Geometry: final body of the model. Coordinates: model frame, mm. A direction names the side the tool comes from. Give positions to 0.01 mm unless a question says otherwise; leave off trailing zeros. Write each loop counter-clockwise with the first axis right and the second up, starting at its lowest first coordinate (ties: lowest second). Pieces come first, ordered by that corner, then holes.
from build123d import *

# Parameters (mm, degrees)
BOSS_EXTRU_1_DEPTH      = 5
BOSS_EXTRU_2_DEPTH      = 5
ESQUISSE3_R             = 4
ENL_V_MAT_EXTRU_1_DEPTH = 5


with BuildPart() as part:
    # Esquisse1 → Boss.-Extru.1 (new body)
    with BuildSketch(Plane.XY):
        with BuildLine():
            Line((16.587839799, 53.843180126), (-35.88556985, 8.175453138))
            ThreePointArc((-35.88556985, 8.175453138), (-31.864665417, -54.486574909), (27.523708309, -34.097398918))
            Line((27.523708309, -34.097398918), (49.496452515, 31.904105008))
            ThreePointArc((49.496452515, 31.904105008), (41.417346329, 55.43644284), (16.587839799, 53.843180126))
        make_face()
        with BuildLine():
            Line((23.152792246, 46.299878504), (-29.320617403, 0.632151516))
            ThreePointArc((-29.320617403, 0.632151516), (-26.31766346, -46.166071962), (18.035678944, -30.938712678))
            Line((18.035678944, -30.938712678), (40.008423149, 35.062791248))
            ThreePointArc((40.008423149, 35.062791248), (35.870344371, 47.115939894), (23.152792246, 46.299878504))
        make_face(mode=Mode.SUBTRACT)
    extrude(amount=BOSS_EXTRU_1_DEPTH)

    # Esquisse2 → Boss.-Extru.2 (add)
    with BuildSketch(Plane.XY.offset(5)):
        with BuildLine():
            Line((16.587839799, 53.843180126), (-35.88556985, 8.175453138))
            ThreePointArc((-35.88556985, 8.175453138), (-31.864665417, -54.486574909), (27.523708309, -34.097398918))
            Line((27.523708309, -34.097398918), (49.496452515, 31.904105008))
            ThreePointArc((49.496452515, 31.904105008), (41.417346329, 55.43644284), (16.587839799, 53.843180126))
        make_face()
    extrude(amount=BOSS_EXTRU_2_DEPTH)

    # Esquisse3 → Enlèv. mat.-Extru.1 (cut)
    with BuildSketch(Plane.XY.offset(10)):
        with Locations((-9.954007684, -21.62058827)):
            Circle(ESQUISSE3_R)
    extrude(amount=-ENL_V_MAT_EXTRU_1_DEPTH, mode=Mode.SUBTRACT)


solid = part.part
Q1. Ray query, line 1 along Y through (x, z) = (14, 3); line 2 along Y through (x, z) = (9.5, 3.25); line 3 along X through (y, z) = (19, 3.75). Return the intervals inside material, ascending.
Filled sheet:
line 1: y = -53.03 to -38.84, 38.33 to 51.59
line 2: y = -56 to -43.8, 34.42 to 47.67
line 3: x = -23.45 to -8.22, 34.66 to 45.2
Q2. Section C-C on x = -18. Output: boundary loops of the cut face in (y, z), plus the area to 3 significant figures.
Filled sheet:
outline: (-60.29, 0) - (-50, 0) - (-50, 5) - (10.48, 5) - (10.48, 0) - (23.74, 0) - (23.74, 10) - (-60.29, 10) - close
area: 538 mm2
Q3. Pull-direction query (X, two-part tool) for faces 1 (the flat face through (-9.28, 31.33, 4.93)), 2 (the cylindrical face through (-32.703, -53.912, 4.93)), 3 (the cylindrical face through (-26.94, -45.74, 2.46)), 4 (the flat face through (0, 0, 5)); classes: released by +X, released by -X, zero draft, split by the parting line, or undercut.
Filled sheet:
face 1: released by -X
face 2: split by the parting line
face 3: undercut
face 4: undercut
Q4. Section B-B on y = -5. Output: boundary loops of the cut face in (x, z), plus the area to 3 significant figures.
Filled sheet:
outline: (-45.79, 0) - (-34.33, 0) - (-34.33, 5) - (26.67, 5) - (26.67, 0) - (37.21, 0) - (37.21, 10) - (-45.79, 10) - close
area: 525 mm2
Q5. Section A-A on z = 3.5. Output: boundary loops of the cut face in (x, y), plus the area to 3 significant figures.
Filled sheet:
outline: (-35.89, 8.18) arc R39.5 ccw (long way) to (27.52, -34.1) - (49.5, 31.9) arc R20.5 ccw to (16.59, 53.84) - close; hole (-29.32, 0.63) arc R29.5 ccw (long way) to (18.04, -30.94) - (40.01, 35.06) arc R10.5 ccw to (23.15, 46.3) - close
area: 3,060 mm2
Q6. Access query for faces 5 (the flat face through (-2.7, 23.8, 2.5)), 6 (the cylindrical face through (-6.14, -20.42, 7.54)). Directions: +Z, -Z, +X, -X, +Y, -Y. A direction counts if a zero-diameter tool reaches every point of the face in a straight line with its end or side. Return the directions, or none.
Filled sheet:
face 5: -Z
face 6: +Z, -Z
Q7. Pin query (flat end, axial travel): P1, Ø1.5, axis at x = 2.5, z = 5.5, coming from the -Y side; P2, Ø1, axis at x = -35.5, z = 4.5, coming from the -Y side; P3, Ø12, axis at x = -23, y = -8.5, coming from the -Z side; P4, Ø10, axis at x = 26, y = -11, coming from the -Z side. Return the tip coordinate at first contact, or that it passes through.
Filled sheet:
P1: stops at y = -59.35
P2: stops at y = -52.16
P3: stops at z = 5
P4: stops at z = 0
